Design review of the part shown in the three views and the two pictorial views. Dimensions are in mm from the part's minimum x, y and z. A direction names the side the tool comes from. Give positions to 0.01 mm unless a question says otherwise; leave off trailing zeros. Order: outer loops, then holes, each group sorted by start corner. A loop starts at its lowest first (then second) coordinate and runs counter-clockwise, first axis right, second up.
Item 1: The part is to be moulded in two halves that separate along Y. For the marked faces 1, 2, 3 and 4, say which applies: released by +Y, released by -Y, zero draft, split by the parting line, or undercut.
Item 2: Consider section A-A (y = 12). Give the boundary of the cut face in (x, z), plus the area to 3 significant figures.
Item 3: Consider section C-C (x = 5). Give the boundary of the cut face in (y, z), plus the area to 3 significant figures.
Item 4: Consider section D-D (x = 22.5). Give the boundary of the cut face in (y, z), plus the area to 3 significant figures.
Item 5: For probe 1 along Y at (x, z) = (22.5, 2.4); probe 2 along X at (y, z) = (11, 5.45); probe 3 along Y at (x, z) = (40, 3.9), list the stretches that pass through material, from the lowest coordinate up.
Item 6: Consider section B-B (z = 4.45). Give the boundary of the cut face in (x, y).
Item 7: For P1, Ø1.5, axis at y = 3, z = 5, coming from the +X side; P2, Ø0.9, axis at x = 40, z = 4.5, coming from the -Y side; P3, Ø4.5, axis at x = 5, y = 12, coming from the -Z side, all flat-tipped, find the tip position at first contact; note any pin that passes through.
Item 8: Machinability: for the marked faces 5, 6, 7, 8 and 9, which of the approach directions +Z, -Z, +X, -X, +Y, -Y give a long, thin tool a straight path to every point of the face, cutting with its end or side? Answer none if there is none.
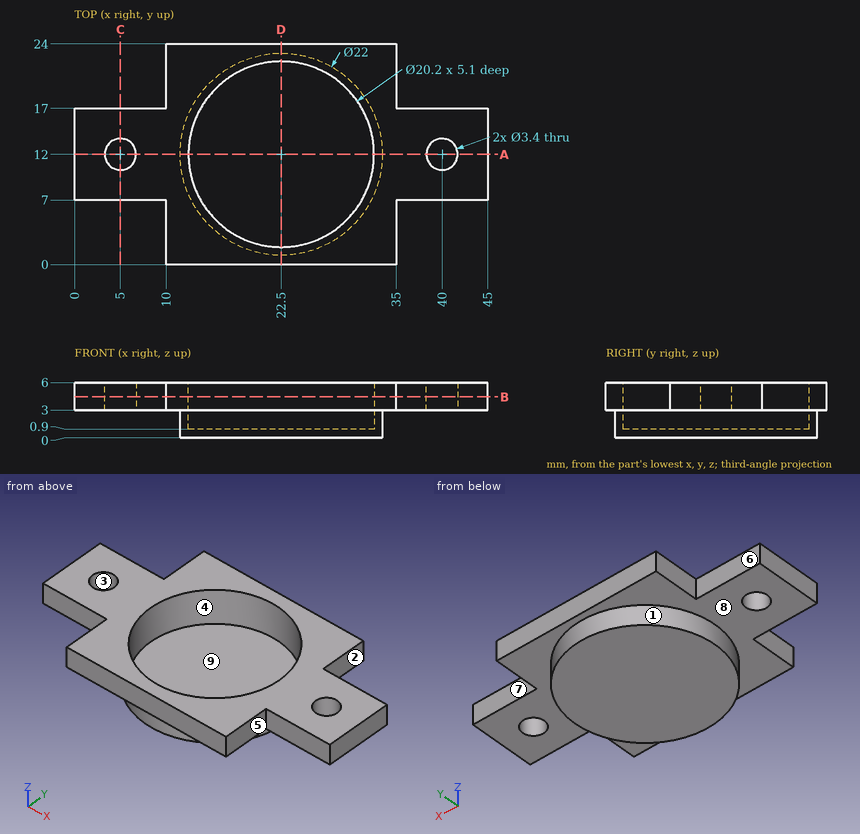
Resolved:
1. face 1: split by the parting line
1. face 2: zero draft
1. face 3: undercut
1. face 4: undercut
2. outline: (0, 3) - (3.3, 3) - (3.3, 6) - (0, 6) - close; (6.7, 3) - (11.5, 3) - (11.5, 0) - (33.5, 0) - (33.5, 3) - (38.3, 3) - (38.3, 6) - (32.6, 6) - (32.6, 0.9) - (12.4, 0.9) - (12.4, 6) - (6.7, 6) - close; (41.7, 3) - (45, 3) - (45, 6) - (41.7, 6) - close
2. area: 77.6 mm2
3. outline: (7, 3) - (10.3, 3) - (10.3, 6) - (7, 6) - close; (13.7, 3) - (17, 3) - (17, 6) - (13.7, 6) - close
3. area: 19.8 mm2
4. outline: (0, 3) - (1, 3) - (1, 0) - (23, 0) - (23, 3) - (24, 3) - (24, 6) - (22.1, 6) - (22.1, 0.9) - (1.9, 0.9) - (1.9, 6) - (0, 6) - close
4. area: 35.0 mm2
5. probe 1: y = 1 to 1.9, 22.1 to 23
5. probe 2: x = 0 to 3.63, 6.37 to 12.45, 32.55 to 38.63, 41.37 to 45
5. probe 3: y = 7 to 10.3, 13.7 to 17
6. outline: (0, 7) - (10, 7) - (10, 0) - (35, 0) - (35, 7) - (45, 7) - (45, 17) - (35, 17) - (35, 24) - (10, 24) - (10, 17) - (0, 17) - close; hole circle Ø3.4 at (5, 12); hole circle Ø20.2 at (22.5, 12); hole circle Ø3.4 at (40, 12)
7. P1: stops at x = 35
7. P2: stops at y = 7
7. P3: stops at z = 3
8. face 5: +Z, -Z, +X, -Y
8. face 6: +Z, -Z, -X, +Y
8. face 7: +Z, -Z, +X, +Y
8. face 8: -Z
8. face 9: +Z
